Source: three-view drawing plus pictorial views. Frame: mm from the lowest corner of the part. Coordinates: 2 decimals unless noted, no trailing zeros. Write each loop counter-clockwise with the first axis right and the second up, starting at its lowest first coordinate (ties: lowest second). Pieces come first, ordered by that corner, then holes. Notation, with made-up numbers: (31, 67) - (66, 67) arc R8 ccw to (66, 74) - close; hole circle Ø11 at (60.5, 29). An arc over 180 degrees is marked (long way). One line per item, written item: value.
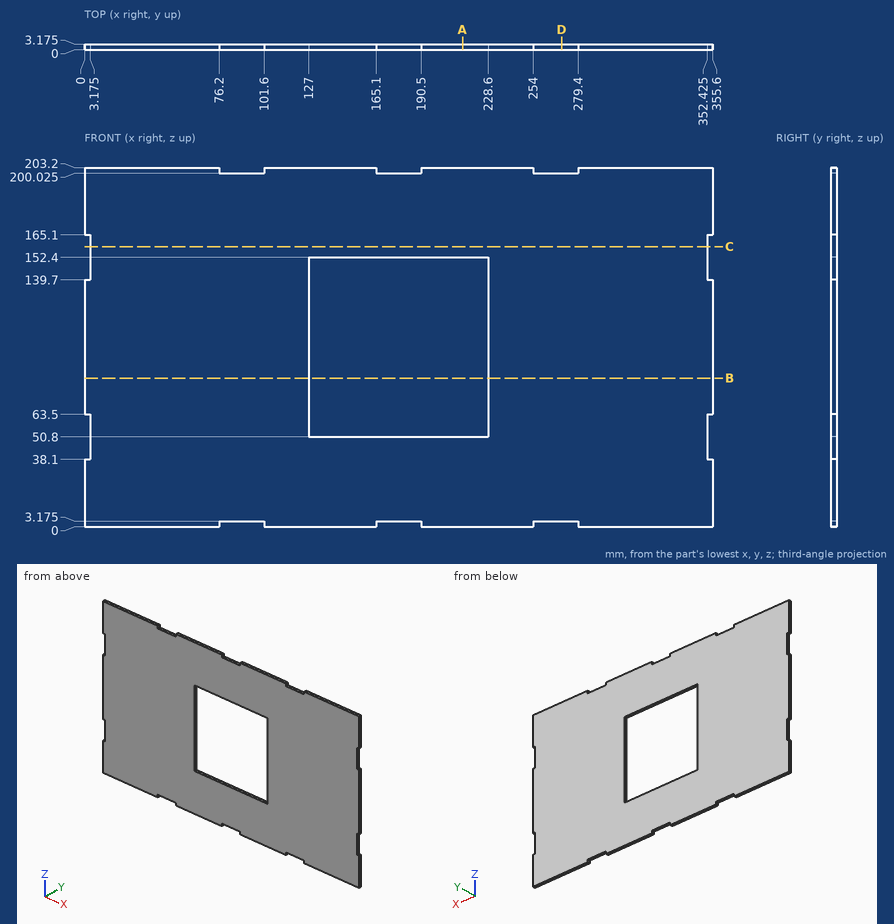
1) Material intervals for line 1 (X direction, y = 2.4, z = 89); line 2 (X direction, y = 2.55, z = 54.5) (3 decimals); line 3 (Z direction, x = 190, y = 0.55) (3 decimals), sorted ascending.
Values found:
line 1: 0 to 127, 228.6 to 355.6
line 2: 3.175 to 127, 228.6 to 352.425
line 3: 3.175 to 50.8, 152.4 to 200.025
2) Section query A-A on x = 214. Output: boundary loops of the cut face in (y, z) (3 decimals), then the cut area to 3 significant figures.
Values found:
outline: (0, 0) - (3.175, 0) - (3.175, 50.8) - (0, 50.8) - close; (0, 152.4) - (3.175, 152.4) - (3.175, 203.2) - (0, 203.2) - close
area: 323 mm2
3) Contact query for flat-ended pins moving along their axis: P1, Ø1.6, axis at x = 171.5, y = 1.5, coming from the +Z side (3 decimals); P2, Ø1, axis at y = 1, z = 50.5, coming from the -X side (3 decimals). Output: stop coordinate, or through.
Values found:
P1: z = 200.025
P2: x = 3.175
4) Section query D-D on x = 270. Output: boundary loops of the cut face in (y, z) (3 decimals).
Values found:
outline: (0, 3.175) - (3.175, 3.175) - (3.175, 200.025) - (0, 200.025) - close
5) Section query B-B on z = 84. Output: boundary loops of the cut face in (x, y) (3 decimals), then the cut area to 3 significant figures.
Values found:
outline: (0, 0) - (127, 0) - (127, 3.175) - (0, 3.175) - close; (228.6, 0) - (355.6, 0) - (355.6, 3.175) - (228.6, 3.175) - close
area: 806 mm2
6) Section query C-C on z = 158.5. Output: boundary loops of the cut face in (x, y) (3 decimals).
Values found:
outline: (3.175, 0) - (352.425, 0) - (352.425, 3.175) - (3.175, 3.175) - close
